Check sheet for the modelled part. Datum: model origin and axes. Units: mm. A direction names the side the tool comes from. Coordinates: 2 decimals unless noted, no trailing zeros. Loops run counter-clockwise (first coordinate to the right, second up) from the corner with the lowest first, then second, coordinate; pieces in that order, holes last. Notation, with made-up numbers: (69, -17.75) - (83, -17.75) arc R10 ccw to (83, -9.75) - close; hole circle Ø7 at (-35, 83.5). An arc over 180 degrees is marked (long way). Use a Markdown table: item, result. Add a question column.
1) Sectioned sample at A-A, the plane x = 0. Enter the section's corners in (y, z), then the cut area to 3 significant figures.
2) Go/stop test with flat-tipped pins: P1, Ø1.5, axis at x = -485.5, z = 7.5, coming from the -Y side; P2, Ø5, axis at x = -491, z = 7, coming from the +Y side. Record where each tip stops, or that it passes through.
3) Draft check along Y on faces 1 (the cylindrical face through (2.197, 795.016, 4.93)), 2 (the flat face through (688.509, 1630.396, 4.93)), 3 (the flat face through (-125, 756, 10)). Enter one of: pulls with the +Y half, pulls with the -Y half, needs draft (parallel to the pull), parting line crosses it, or undercut.
4) Tool access check on faces 4 (the flat face through (-792.39, 1535.32, 4.93)), 5 (the cylindrical face through (-3.373, 1104.963, 4.93)). Record the directions out of +Z, -Z, +X, -X, +Y, -Y that give a thin tool (end or side, any length) a straight path to the whole face; none if there is none.
5) Sectioned sample at D-D, the plane x = 756. Enter the section's corners in (y, z), then the cut area to 3 significant figures.
6) Sectioned sample at B-B, the plane y = 151.5. Enter the section's corners in (x, z).
7) Sectioned sample at C-C, the plane z = 3.25. Enter the section's corners in (x, y).
8) Thickness scan on line 1 (Y direction, x = -954.5, z = 8.25); line 2 (Y direction, x = -937, z = 7); line 3 (X direction, y = 813, z = 7.5). Record the ranges inside material, lowest first.
Autodesk Inventor part; units mm, degrees
ref_plane "YZ Plane" through (0, 0, 0) normal (1, 0, 0) x (0, 1, 0)
ref_plane "XZ Plane" through (0, 0, 0) normal (0, 1, 0) x (-1, 0, 0)
ref_plane "XY Plane" through (0, 0, 0) normal (0, 0, 1) x (1, 0, 0)
sketch "Sketch1" plane through (0, 0, 0) normal (0, 0, 1) x (1, 0, 0)
  line L0 (0, 0) -> (0, 1910) construction
  line L1 (424.5155, 1910) -> (-415.4845, 1910)
  line L2 (-415.4845, 1910) -> (-1180, 1150)
  line L3 (-1180, 0) -> (-1180, 1150)
  line L4 (960, 0) -> (960, 1342.8524)
  line L5 (424.5155, 1910) -> (960, 1342.8524)
  circle A0 centre (0, 950) radius 195 construction
  line L6 (960, 0) -> (-1180, 0)
  circle A1 centre (-960, 220) radius 200.5
  circle A2 centre (-588, 255) radius 38
  circle A3 centre (374.6358, 1277) radius 50
  circle A4 centre (0, 950) radius 155
  point P0 (0, 955)
  dimension "d1" = 840
  dimension "d3" = 1150
  dimension "d11" = 390
  dimension "d12" = 1180
  dimension "d13" = 950
  dimension "d14" = 76
  dimension "d15" = 1910
  dimension "d16" = 255
  dimension "d17" = 220
  dimension "d18" = 401
  dimension "d19" = 220
  dimension "d21" = 1277
  dimension "d22" = 1554.6358
  dimension "d23" = 100
  dimension "d33" = 2140
  dimension "d34" = 494
  dimension "d45" = 310
  dimension "d49" = 372
  dimension "d51" = 780
  dimension "d52" = 1078
extrude "Extrusion1" add sketch "Sketch1" along normal blind 10
sketch "Sketch3" plane through (0, 0, 10) normal (0, 0, 1) x (1, 0, 0)
  line L0 (-400, 950) -> (400, 950) construction
  circle A0 centre (0, 950) radius 155
  circle A1 centre (155, 950) radius 2.5
  circle A2 centre (-155, 950) radius 2.5
  line L1 (132.7592, 870) -> (-132.7592, 870) construction
  circle A3 centre (132.7592, 870) radius 2.5
  circle A4 centre (-132.7592, 870) radius 2.5
  point P0 (0, 0)
  point P1 (-154.9798, 947.5001)
  point P2 (-154.9798, 952.4999)
  point P3 (154.9798, 947.5001)
  point P4 (154.9798, 952.4999)
  point P5 (134.0322, 872.1516)
  point P6 (131.4516, 867.8692)
  dimension "d47" = 5
  dimension "d48" = 80
extrude "Extrusion3" cut sketch "Sketch3" against normal through all contours A0 A1 | A0 A2 | A3 A0 | A4 A0 | A0 A4 picked at (155.7492, 949.3589) picked at (-155.8257, 950.101) picked at (133.5004, 869.6223)
equation "\"d17\" = d19"
properties part number "ДМФ 012 Стенка Нос"
Solved:
| question | item | result |
|---|---|---|
| 1 | outline | (0, 0) - (795, 0) - (795, 10) - (0, 10) - close; (1105, 0) - (1910, 0) - (1910, 10) - (1105, 10) - close |
| 1 | area | 16,000 mm2 |
| 2 | P1 | stops at y = 0 |
| 2 | P2 | stops at y = 1837.42 |
| 3 | face 1 | undercut |
| 3 | face 2 | pulls with the +Y half |
| 3 | face 3 | needs draft |
| 4 | face 4 | +Z, -Z, -X, +Y |
| 4 | face 5 | +Z, -Z |
| 5 | outline | (0, 0) - (1558.91, 0) - (1558.91, 10) - (0, 10) - close |
| 5 | area | 15,600 mm2 |
| 6 | outline | (-1180, 0) - (-1148.44, 0) - (-1148.44, 10) - (-1180, 10) - close; (-771.56, 0) - (960, 0) - (960, 10) - (-771.56, 10) - close |
| 7 | outline | (-1180, 0) - (960, 0) - (960, 1342.85) - (424.52, 1910) - (-415.48, 1910) - (-1180, 1150) - close; hole circle Ø401 at (-960, 220); hole circle Ø76 at (-588, 255); hole (-154.98, 947.5) arc R155 ccw to (-134.03, 872.15) arc R2.5 ccw (long way) to (-131.45, 867.87) arc R155 ccw to (131.45, 867.87) arc R2.5 ccw (long way) to (134.03, 872.15) arc R155 ccw to (154.98, 947.5) arc R2.5 ccw (long way) to (154.98, 952.5) arc R155 ccw to (-154.98, 952.5) arc R2.5 ccw (long way) to start; hole circle Ø100 at (374.64, 1277) |
| 8 | line 1 | y = 0 to 19.58, 420.42 to 1374.17 |
| 8 | line 2 | y = 0 to 20.82, 419.18 to 1391.56 |
| 8 | line 3 | x = -1180 to -72.5, 72.5 to 960 |
